```python
from build123d import *

# Parameters (mm, degrees)
F0_W     = 254
F0_H     = 254
F1_DEPTH = 203.2
F1_TAPER = 5
F2_SIZE  = 25.4
F4_DEPTH = 38.1


with BuildPart() as f1:
    # F0 (on Top) → F1 (new body)
    with BuildSketch(Plane.XY):
        Rectangle(F0_W, F0_H)
    extrude(amount=F1_DEPTH, taper=F1_TAPER)

    # F2
    f2_edges = [f1.edges().sort_by_distance(p)[0] for p in [
        (-118.111152, -118.111152, 101.6),
        (118.111152, -118.111152, 101.6),
        (118.111152, 118.111152, 101.6),
        (-118.111152, 118.111152, 101.6),
    ]]
    chamfer(f2_edges, length=F2_SIZE)

    # F3 (on face) → F4 (cut)
    with BuildSketch(Plane.XY.offset(203.2)):
        Polygon((19.05, 44.45), (19.05, 132.0214867592), (-19.05, 132.0214867592), (-19.05, 44.45), (-44.45, 44.45), (-44.45, 19.05), (-137.8337591887, 19.05), (-137.8337591887, -19.05), (-44.45, -19.05), (-44.45, -44.45), (-19.05, -44.45), (-19.05, -130.3608417511), (19.05, -130.3608417511), (19.05, -44.45), (44.45, -44.45), (44.45, -19.05), (136.5052312613, -19.05), (136.5052312613, 19.05), (44.45, 19.05), (44.45, 44.45), align=None)
    extrude(amount=-F4_DEPTH, mode=Mode.SUBTRACT)


solid = f1.part
```
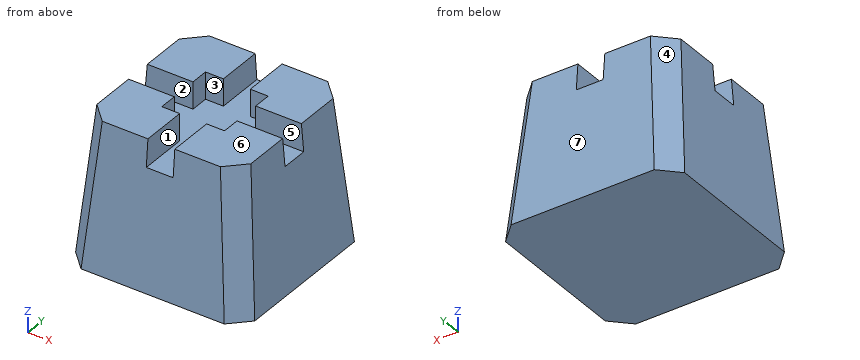
Check sheet for the modelled part. Datum: model origin and axes. Units: mm. Face numbers are marked on the shaded views. A direction names the side the tool comes from. Round coordinates to 2 decimals unless told otherwise and drop trailing zeros. Order: outer loops, then holes, each group sorted by start corner. A loop starts at its lowest first (then second) coordinate and runs counter-clockwise, first axis right, second up. Notation, with made-up numbers: (66.5, 64.5) -> (78.5, 64.5) arc R22 cw to (78.5, 74.5) -> close; hole circle Ø11 at (-27, -27). An arc over 180 degrees is marked (long way). One line per item, written item: value. Start each with the question number.
Q1. Gauge pin test, flat ends, axial feed: pin 1 Ø11.5 at (x, z) = (76.5, 181.5) entering from -Y; pin 2 Ø3 at (x, z) = (-53, 126.5) entering from +Y; pin 3 Ø1.5 at (x, z) = (-17, 48) entering from -Y. Record the tip position at first contact, or that the pin passes through.
Q2. Cross-section at C-C (z = 173). Record the boundary of the cut face in (x, y).
Q3. Cross-section at D-D (y = 92.5). Record the boundary of the cut face in (x, z).
Q4. Thickness scan on line 1 (Y direction, x = -74.5, z = 166); line 2 (Z direction, x = 18, y = -108.5); line 3 (Y direction, x = -83, z = 187). Record the ranges inside material, lowest first.
Q5. Set-up check for the marked faces 1, 2, 3 and 4: record each of +Z, -Z, +X, -X, +Y, -Y from which the full face is reachable in a straight line by a thin tool's end or side.
Q6. Mould release check, pull along Y, two halves, no side actions. Record for the marked faces 5, 6 and 7: pulls with the +Y half, pulls with the -Y half, needs draft (parallel to the pull), parting line crosses it, or undercut.
Q7. Cross-section at A-A (x = 61.5). Record the boundary of the cut face in (y, z).
Completed:
1. pin 1: stops at y = -111.62
1. pin 2: stops at y = 116.06
1. pin 3: stops at y = -122.87
2. outline: (-111.86, -86.37) -> (-86.37, -111.86) -> (-19.05, -111.86) -> (-19.05, -44.45) -> (-44.45, -44.45) -> (-44.45, -19.05) -> (-111.86, -19.05) -> close; (-111.86, 19.05) -> (-44.45, 19.05) -> (-44.45, 44.45) -> (-19.05, 44.45) -> (-19.05, 111.86) -> (-86.37, 111.86) -> (-111.86, 86.37) -> close; (19.05, -111.86) -> (86.37, -111.86) -> (111.86, -86.37) -> (111.86, -19.05) -> (44.45, -19.05) -> (44.45, -44.45) -> (19.05, -44.45) -> close; (19.05, 44.45) -> (44.45, 44.45) -> (44.45, 19.05) -> (111.86, 19.05) -> (111.86, 86.37) -> (86.37, 111.86) -> (19.05, 111.86) -> close
3. outline: (-127, 0) -> (127, 0) -> (118, 102.91) -> (100.45, 203.2) -> (19.05, 203.2) -> (19.05, 165.1) -> (-19.05, 165.1) -> (-19.05, 203.2) -> (-100.45, 203.2) -> (-118, 102.91) -> close
4. line 1: y = -112.48 to -19.05, 19.05 to 112.48
4. line 2: z = 0 to 165.1
4. line 3: y = -110.64 to -19.05, 19.05 to 110.64
5. face 1: +Z, +Y, -Y
5. face 2: +Z, +X, -X
5. face 3: +Z
5. face 4: +Z, -X, +Y
6. face 5: undercut
6. face 6: needs draft
6. face 7: pulls with the +Y half
7. outline: (-127, 0) -> (127, 0) -> (109.22, 203.2) -> (19.05, 203.2) -> (19.05, 165.1) -> (-19.05, 165.1) -> (-19.05, 203.2) -> (-109.22, 203.2) -> close
